Answer from the drawing. Dimensions are ordinates in mm from the lowest x, y and z of the part. A direction names the side the tool comes from. Round coordinates to 2 decimals unless told otherwise and drop trailing zeros. Loops run counter-clockwise (first coordinate to the right, second up) from the corner with the lowest first, then second, coordinate; pieces in that order, holes last. Notation, with made-up numbers: (51, 45.25) - (96, 45.25) arc R23 ccw to (96, 63.25) - close; hole circle Ø11 at (67, 16.25). An arc over 180 degrees is marked (long way). Return JSON: item names as keys, results as strings.
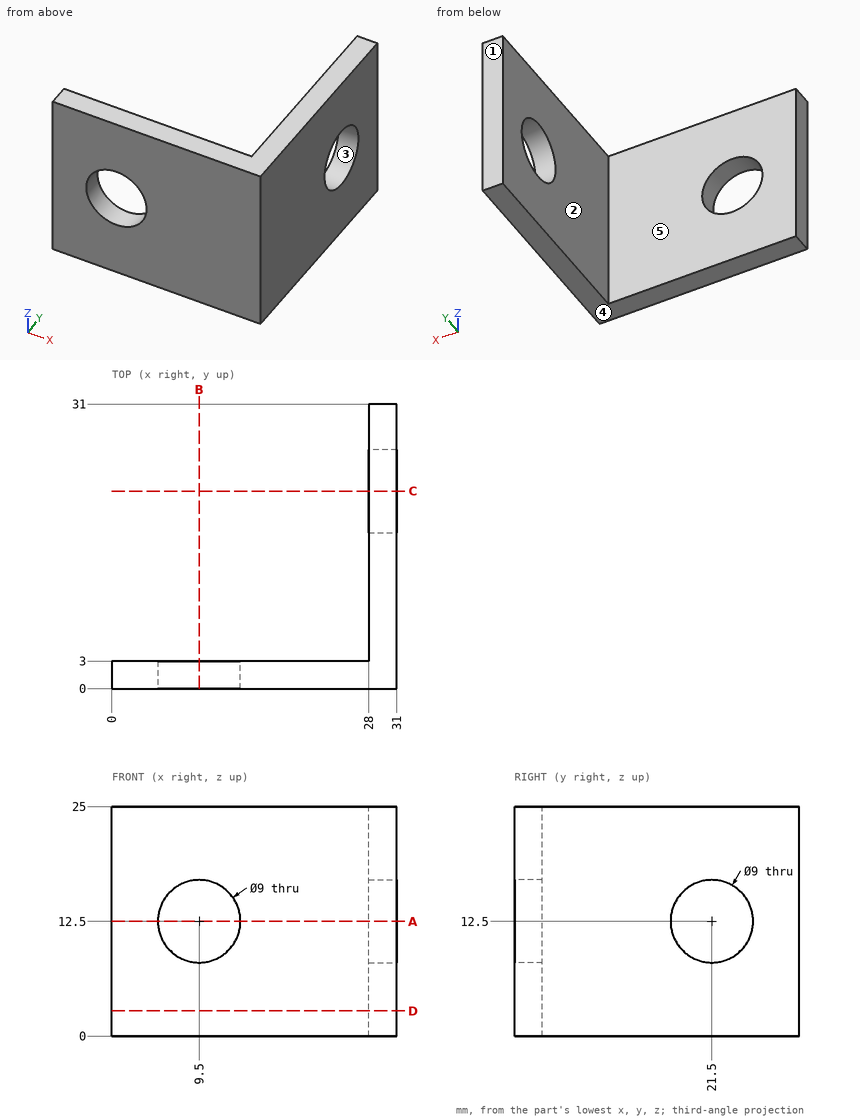
1) Find the intervals of material crossed by L1, parallel to Z at x = 9.5, y = 2.25; L2, parallel to X at y = 11, z = 6.25; L3, parallel to Y at x = 11.5, z = 4.5, in increasing order.
Verdict:
{"L1": "z = 0 to 8, 17 to 25", "L2": "x = 28 to 31", "L3": "y = 0 to 3"}
2) Section D-D (z = 2.75) is taken. Give the vertices of the cut face in (x, y).
Verdict:
{"outline": "(0, 0) - (31, 0) - (31, 31) - (28, 31) - (28, 3) - (0, 3) - close"}
3) A tool of negligible diameter and unlimited length cuts with its end or side. For the marked faces 1 and 2, from which of +Z, -Z, +X, -X, +Y, -Y can it reach the whole face along a straight path? Write none if from no direction.
Verdict:
{"face 1": "+Z, -Z, +X, -X, +Y", "face 2": "+Z, -Z, -X, +Y"}
4) Flat-ended cylindrical pins translate along their axes: pin 1 (12 mm diameter, centred on x = 13.5, y = 12.5, fed in from +Z); pin 2 (7.5 mm diameter, centred on y = 12.5, z = 16.5, fed in from -X); pin 3 (6 mm diameter, centred on x = 7.5, z = 10.5, fed in from +Y). Find the tip coordinate at first contact, or state that the pin passes through.
Verdict:
{"pin 1": "passes through", "pin 2": "stops at x = 28", "pin 3": "stops at y = 3"}
5) Section B-B (x = 9.5) is taken. Give the vertices of the cut face in (y, z), and give its area (3 significant figures).
Verdict:
{"outline": "(0, 0) - (3, 0) - (3, 8) - (0, 8) - close; (0, 17) - (3, 17) - (3, 25) - (0, 25) - close", "area": "48.0 mm2"}
6) Section A-A (z = 12.5) is taken. Give the vertices of the cut face in (x, y), and give its area (3 significant figures).
Verdict:
{"outline": "(0, 0) - (5, 0) - (5, 3) - (0, 3) - close; (14, 0) - (31, 0) - (31, 17) - (28, 17) - (28, 3) - (14, 3) - close; (28, 26) - (31, 26) - (31, 31) - (28, 31) - close", "area": "123 mm2"}
7) Determine the mould class of the marked faces 3, 4 and 5 for opening direction Z: pulls with the +Z half, pulls with the -Z half, needs draft (parallel to the pull), parting line crosses it, or undercut.
Verdict:
{"face 3": "undercut", "face 4": "pulls with the -Z half", "face 5": "needs draft"}
8) Section C-C (y = 21.5) is taken. Give the vertices of the cut face in (x, z), and give its area (3 significant figures).
Verdict:
{"outline": "(28, 0) - (31, 0) - (31, 8) - (28, 8) - close; (28, 17) - (31, 17) - (31, 25) - (28, 25) - close", "area": "48.0 mm2"}
